Verification items for the finished model (mm, model axes). A direction names the side the tool comes from. Round coordinates to 2 decimals unless told otherwise and drop trailing zeros. Write each loop counter-clockwise with the first axis right and the second up, starting at its lowest first coordinate (ties: lowest second). Pieces come first, ordered by that corner, then holes.
from build123d import *

# Parameters (mm, degrees)
SKETCH_W     = 9.91
SKETCH_H     = 11.43
PAD_DEPTH    = 7.62
SKETCH002_W  = 0.64
SKETCH002_H  = 0.64
SKETCH004_W  = 0.64
SKETCH004_H  = 0.64
SKETCH006_W  = 0.64
SKETCH006_H  = 0.64
SKETCH008_W  = 0.64
SKETCH008_H  = 0.64
POCKET_DEPTH = 11.431
SKETCH010_W  = 6.35
SKETCH010_H  = 9.525
PAD001_DEPTH = 4.19
CHAMFER_SIZE = 1


with BuildPart() as part:
    # Sketch → Pad (new body)
    with BuildSketch(Plane.XZ):
        with Locations((0, 5.715)):
            Rectangle(SKETCH_W, SKETCH_H)
    extrude(amount=-PAD_DEPTH)

    # AdditivePipe: sweep along a path in Sketch001
    with BuildLine(Plane.YZ) as additivepipe_path:
        Line((0, 9.525), (8.942893, 9.525))
        ThreePointArc((8.942893, 9.525), (9.325577, 9.44888), (9.65, 9.232107))
        Line((9.65, 9.232107), (16.977107, 1.905))
        ThreePointArc((16.977107, 1.905), (17.19388, 1.580577), (17.27, 1.197893))
        Line((17.27, 1.197893), (17.27, -3.68))
    # Sketch002 → AdditivePipe (sweep)
    with BuildSketch(Plane.XZ):
        with Locations((3.81, 9.525)):
            Rectangle(SKETCH002_W, SKETCH002_H)
    additivepipe = sweep(path=additivepipe_path.line)

    # AdditivePipe001: sweep along a path in Sketch003
    with BuildLine(Plane.YZ) as additivepipe001_path:
        Line((0, 6.985), (8.942893, 6.985))
        ThreePointArc((8.942893, 6.985), (9.325577, 6.90888), (9.65, 6.692107))
        Line((9.65, 6.692107), (14.437107, 1.905))
        ThreePointArc((14.437107, 1.905), (14.65388, 1.580577), (14.73, 1.197893))
        Line((14.73, 1.197893), (14.73, -3.68))
    # Sketch004 → AdditivePipe001 (sweep)
    with BuildSketch(Plane.XZ):
        with Locations((3.81, 6.985)):
            Rectangle(SKETCH004_W, SKETCH004_H)
    additivepipe001 = sweep(path=additivepipe001_path.line)

    # AdditivePipe002: sweep along a path in Sketch005
    with BuildLine(Plane.YZ) as additivepipe002_path:
        Line((0, 4.445), (8.942893, 4.445))
        ThreePointArc((8.942893, 4.445), (9.325577, 4.36888), (9.65, 4.152107))
        Line((9.65, 4.152107), (11.897107, 1.905))
        ThreePointArc((11.897107, 1.905), (12.11388, 1.580577), (12.19, 1.197893))
        Line((12.19, 1.197893), (12.19, -3.68))
    # Sketch006 → AdditivePipe002 (sweep)
    with BuildSketch(Plane.XZ):
        with Locations((3.81, 4.445)):
            Rectangle(SKETCH006_W, SKETCH006_H)
    additivepipe002 = sweep(path=additivepipe002_path.line)

    # AdditivePipe003: sweep along a path in Sketch007
    with BuildLine(Plane.YZ) as additivepipe003_path:
        Line((0, 1.905), (8.65, 1.905))
        ThreePointArc((8.65, 1.905), (9.357107, 1.612107), (9.65, 0.905))
        Line((9.65, 0.905), (9.65, -3.68))
    # Sketch008 → AdditivePipe003 (sweep)
    with BuildSketch(Plane.XZ):
        with Locations((3.81, 1.905)):
            Rectangle(SKETCH008_W, SKETCH008_H)
    additivepipe003 = sweep(path=additivepipe003_path.line)

    # Mirrored: AdditivePipe, AdditivePipe001, AdditivePipe002, AdditivePipe003 across Sketch002 V_Axis
    add(additivepipe.mirror(Plane(origin=(0, 0, 0), x_dir=(0, -1, 0), z_dir=(1, 0, 0))))
    add(additivepipe001.mirror(Plane(origin=(0, 0, 0), x_dir=(0, -1, 0), z_dir=(1, 0, 0))))
    add(additivepipe002.mirror(Plane(origin=(0, 0, 0), x_dir=(0, -1, 0), z_dir=(1, 0, 0))))
    add(additivepipe003.mirror(Plane(origin=(0, 0, 0), x_dir=(0, -1, 0), z_dir=(1, 0, 0))))

    # Sketch009 (on Face3 of AdditivePipe002) → Pocket (cut, through all)
    with BuildSketch(Plane(origin=(0, 0, 0), x_dir=(1, 0, 0), z_dir=(0, 0, -1))):
        Polygon((-4.955, 0), (4.955, 0), (4.366103, -1.02), (-4.366103, -1.02), align=None)
    extrude(amount=-POCKET_DEPTH, mode=Mode.SUBTRACT)

    # Sketch010 (on Face7 of Pocket) → Pad001 (join)
    with BuildSketch(Plane.XZ.offset(-1.02)):
        with Locations((0, 5.715)):
            Rectangle(SKETCH010_W, SKETCH010_H)
    extrude(amount=PAD001_DEPTH)

    # Chamfer
    chamfer_edges = [part.edges().sort_by_distance(p)[0] for p in [
        (-4.955, 3.81, 11.43),
    ]]
    chamfer(chamfer_edges, length=CHAMFER_SIZE)


solid = part.part
Q1. Sectioned sample at A-A (z = 3). Give the number of separate pieces and of enclosed holes in the cut face, plus the area to 3 significant figures.
Recorded:
separate pieces: 7
enclosed holes: 0
area: 96.1 mm2
Q2. Sectioned sample at B-B (y = 11.25). Enter the section's corners in (x, z), plus the area to 3 significant figures.
Recorded:
outline: (-4.13, 2.1) - (-3.49, 2.1) - (-3.49, 3) - (-4.13, 3) - close; (-4.13, 4.64) - (-3.49, 4.64) - (-3.49, 5.54) - (-4.13, 5.54) - close; (-4.13, 7.18) - (-3.49, 7.18) - (-3.49, 8.08) - (-4.13, 8.08) - close; (3.49, 2.1) - (4.13, 2.1) - (4.13, 3) - (3.49, 3) - close; (3.49, 4.64) - (4.13, 4.64) - (4.13, 5.54) - (3.49, 5.54) - close; (3.49, 7.18) - (4.13, 7.18) - (4.13, 8.08) - (3.49, 8.08) - close
area: 3.48 mm2
Q3. Material ranges on line 1 along X through (y, z) = (14.5, -1.5); line 2 along X through (y, z) = (-0.5, 10) (3 decimals); line 3 along Z through (x, y) = (-3, 2.5), recorded low to high.
Recorded:
line 1: x = -4.13 to -3.49, 3.49 to 4.13
line 2: x = -3.175 to 3.175
line 3: z = 0 to 11.43
Q4. Depth check by flat-ended pin: P1, Ø1.5, axis at y = 12.5, z = 3.5, coming from the +X side; P2, Ø2, axis at x = -2.5, y = 0.5, coming from the +Z side; P3, Ø5, axis at x = -2, z = 7, coming from the +Y side. Enter the tip coordinate at first touch or a pass-through.
Recorded:
P1: stops at x = 4.13
P2: stops at z = 11.43
P3: stops at y = 14.34
Q5. Release check for a two-part mould opening along X. For faces 6 (the flat face through (-4.656, 0.517, 5.432)), 7 (the flat face through (0, -3.17, 6)), 8 (the flat face through (-4.13, 12, 2)), 9 (the flat face through (4.955, 4, 6)) record: released by +X, released by -X, zero draft, split by the parting line, or undercut.
Recorded:
face 6: undercut
face 7: zero draft
face 8: released by -X
face 9: released by +X
Q6. Tool access check on faces 1 (the flat face through (3.175, -1, 6)), 2 (the flat face through (4.13, 12, 2)), 3 (the flat face through (3.49, 9.6, 0)), 4 (the flat face through (0, -1, 0.952)), 5 (the flat face through (3.81, 13.14, 5.29)). Record the directions out of +Z, -Z, +X, -X, +Y, -Y that give a thin tool (end or side, any length) a straight path to the whole face; none if there is none.
Recorded:
face 1: +Z, -Z, -Y
face 2: +Z, -Z, +X, +Y
face 3: +Z, -Z, +Y
face 4: -Z, -Y
face 5: +X, -X
Q7. Sectioned sample at C-C (x = -2.25). Enter the section's corners in (y, z).
Recorded:
outline: (-3.17, 0.95) - (1.02, 0.95) - (1.02, 0) - (7.62, 0) - (7.62, 11.43) - (1.02, 11.43) - (1.02, 10.48) - (-3.17, 10.48) - close
